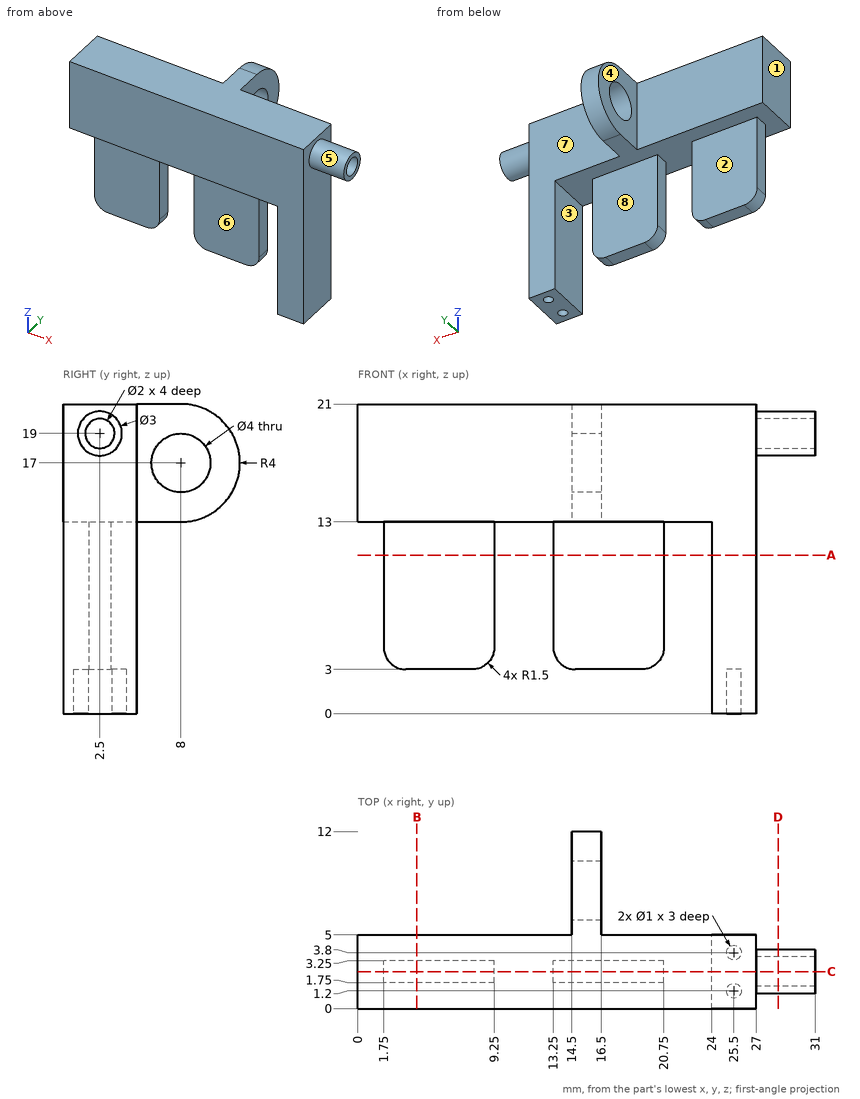
Verification items for this drawing (mm, ordinates from the low corner). A direction names the side the tool comes from. Give positions to 0.01 mm unless a question says otherwise; leave off trailing zeros. Loops run counter-clockwise (first coordinate to the right, second up) from the corner with the lowest first, then second, coordinate; pieces in that order, holes last. Notation, with made-up numbers: M 77.25,85.25 L 92.25,85.25 A13 cw 92.25,94.25 Z; hole C -31.5,25 d4. An arc over 180 degrees is marked long. Return JSON: item names as keys, results as strings. Group by question number.
1. Mould release check, pull along X, two halves, no side actions. Record for the marked faces 1, 2 and 3: released by +X, released by -X, zero draft, split by the parting line, or undercut.
2. Thickness scan on L1, parallel to X at y = 2, z = 9.25; L2, parallel to Y at x = 25.5, z = 1.65; L3, parallel to Y at x = 29.05, z = 19. Record the ranges inside material, lowest first.
3. Tool access check on the marked faces 4, 5, 6, 7 and 8. Record the directions out of +Z, -Z, +X, -X, +Y, -Y that give a thin tool (end or side, any length) a straight path to the whole face; none if there is none.
4. Cross-section at C-C on y = 2.5. Record the boundary of the cut face in (x, z).
5. Cross-section at D-D on x = 28.5. Record the boundary of the cut face in (y, z).
6. Cross-section at B-B on x = 4. Record the boundary of the cut face in (y, z), plus the area to 3 significant figures.
7. Cross-section at A-A on z = 10.75. Record the boundary of the cut face in (x, y).
8. Go/stop test with flat-tipped pins: pin 1 (3 mm diameter, centred on x = 25.5, z = 12.5, fed in from +Y); pin 2 (1 mm diameter, centred on y = 1.5, z = 15, fed in from +X); pin 3 (1.5 mm diameter, centred on x = 27.5, y = 7.5, fed in from -Z); pin 4 (2 mm diameter, centred on x = 18, z = 10, fed in from -Y). Record where each tip stops, or that it passes through.
Return value:
{
 "1": {"face 1": "released by -X", "face 2": "zero draft", "face 3": "undercut"},
 "2": {"L1": "1.75 to 9.25, 13.25 to 20.75, 24 to 27", "L2": "0 to 0.7, 1.7 to 3.3, 4.3 to 5", "L3": "1 to 1.5, 3.5 to 4"},
 "3": {"face 4": "+Z, -Z, -X, +Y", "face 5": "+X", "face 6": "-Z, -X, -Y", "face 7": "+Z, -Z, +X, +Y", "face 8": "-Z, -X, +Y"},
 "4": {"outline": "M 0,13 L 1.75,13 L 1.75,4.5 A1.5 ccw 3.25,3 L 7.75,3 A1.5 ccw 9.25,4.5 L 9.25,13 L 13.25,13 L 13.25,4.5 A1.5 ccw 14.75,3 L 19.25,3 A1.5 ccw 20.75,4.5 L 20.75,13 L 24,13 L 24,0 L 27,0 L 27,17.5 L 31,17.5 L 31,18 L 27,18 L 27,20 L 31,20 L 31,20.5 L 27,20.5 L 27,21 L 0,21 Z"},
 "5": {"outline": "C 2.5,19 d3; hole C 2.5,19 d2"},
 "6": {"outline": "M 0,13 L 1.75,13 L 1.75,3 L 3.25,3 L 3.25,13 L 5,13 L 5,21 L 0,21 Z", "area": "55.0 mm^2"},
 "7": {"outline": "M 1.75,1.75 L 9.25,1.75 L 9.25,3.25 L 1.75,3.25 Z; M 13.25,1.75 L 20.75,1.75 L 20.75,3.25 L 13.25,3.25 Z; M 24,0 L 27,0 L 27,5 L 24,5 Z"},
 "8": {"pin 1": "y = 5", "pin 2": "x = 27", "pin 3": "through", "pin 4": "y = 1.75"}
}
